Autodesk Inventor part; units mm, degrees
ref_plane "YZ Plane" through (0, 0, 0) normal (1, 0, 0) x (0, 1, 0)
ref_plane "XZ Plane" through (0, 0, 0) normal (0, 1, 0) x (-1, 0, 0)
ref_plane "XY Plane" through (0, 0, 0) normal (0, 0, 1) x (1, 0, 0)
sketch "Sketch1" plane through (0, 0, 0) normal (0, 0, 1) x (1, 0, 0)
  line L0 (0, 0) -> (19.05, 0)
  line L1 (19.05, 0) -> (19.05, 24.13)
  line L2 (19.05, 24.13) -> (0, 24.13)
  line L3 (0, 24.13) -> (0, 0)
  dimension "d0" = 19.05
  dimension "d1" = 24.13
extrude "Extrusion1" add sketch "Sketch1" along normal blind 41.275
sketch "Sketch3" plane through (0, 0, 41.275) normal (0, 0, 1) x (1, 0, 0)
  line L0 (19.05, 24.13) -> (0, 24.13)
  line L1 (19.05, 0) -> (11.43, 0)
  line L2 (11.43, 0) -> (11.43, 24.13)
  line L3 (11.43, 24.13) -> (19.05, 24.13)
  line L4 (19.05, 24.13) -> (19.05, 0)
  line L5 (19.05, 0) -> (19.05, 24.13)
  point P0 (0, 0)
  dimension "d4" = 24.13
  dimension "d5" = 0
  dimension "d6" = 7.62
extrude "Extrusion2" add sketch "Sketch3" along normal blind 57.8104
sketch "Sketch4" plane through (11.43, 0, 41.275) normal (-1, 0, 0) x (0, 0, 1)
  line L0 (-41.275, 24.13) -> (57.8104, 24.13)
  line L1 (57.8104, 0) -> (40.1828, 0)
  line L2 (40.1828, 0) -> (40.1828, 24.13)
  line L3 (40.1828, 24.13) -> (57.8104, 24.13)
  line L4 (57.8104, 24.13) -> (57.8104, 0)
  line L5 (57.8104, 24.13) -> (57.8104, 0)
  point P0 (-41.275, 0)
  dimension "d9" = 24.13
  dimension "d10" = 0
  dimension "d11" = 17.6276
extrude "Extrusion3" add sketch "Sketch4" along normal blind 10.16
properties part number "Claw base"
Verification items for the finished model (mm, model axes). A direction names the side the tool comes from. Coordinates: 2 decimals unless noted, no trailing zeros. Order: outer loops, then holes, each group sorted by start corner. A loop starts at its lowest first (then second) coordinate and runs counter-clockwise, first axis right, second up. Notation, with made-up numbers: (43, 71) -> (51, 71) arc R34 cw to (51, 101) -> close; hole circle Ø3 at (20, -26.5). An arc over 180 degrees is marked (long way). Put each result on its own line as item: value. Start each with the question number.
1. Access from +Z, -Z, +X, -X, +Y, -Y to the whole of each face (thin tool, end or side, straight path). Record for faces 1 (the flat face through (6, 12, 81.458)), 2 (the flat face through (1.27, 12, 90)), 3 (the flat face through (12, 0, 50)).
2. Cross-section at D-D, the plane z = 83.5. Record the boundary of the cut face in (x, y).
3. Cross-section at A-A, the plane x = 10.5. Record the boundary of the cut face in (y, z) (3 decimals), then the cut area to 3 significant figures.
4. Material ranges on L1, parallel to Z at x = 9, y = 21 (3 decimals); L2, parallel to X at y = 19.5, z = 59.5, recorded low to high. Write a range as [from, to].
5. Cross-section at B-B, the plane y = 18. Record the boundary of the cut face in (x, z) (3 decimals).
6. Cross-section at C-C, the plane z = 56. Record the boundary of the cut face in (x, y), then the cut area to 3 significant figures.
7. Go/stop test with flat-tipped pins: pin 1 Ø5 at (y, z) = (11.5, 55) entering from -X; pin 2 Ø9 at (y, z) = (10, 87.5) entering from -X. Record where each tip stops, or that it passes through.
Computed:
1. face 1: -X, +Y, -Y
1. face 2: +Z, -X, +Y, -Y
1. face 3: +Z, -Z, +X, -X, -Y
2. outline: (1.27, 0) -> (19.05, 0) -> (19.05, 24.13) -> (1.27, 24.13) -> close
3. outline: (0, 0) -> (24.13, 0) -> (24.13, 41.275) -> (0, 41.275) -> close; (0, 81.458) -> (24.13, 81.458) -> (24.13, 99.085) -> (0, 99.085) -> close
3. area: 1,420 mm2
4. L1: [0, 41.275], [81.458, 99.085]
4. L2: [11.43, 19.05]
5. outline: (0, 0) -> (19.05, 0) -> (19.05, 99.085) -> (1.27, 99.085) -> (1.27, 81.458) -> (11.43, 81.458) -> (11.43, 41.275) -> (0, 41.275) -> close
6. outline: (11.43, 0) -> (19.05, 0) -> (19.05, 24.13) -> (11.43, 24.13) -> close
6. area: 184 mm2
7. pin 1: x = 11.43
7. pin 2: x = 1.27
